Here's how the part is built. I have some questions about the finished solid (model axes, mm). Round coordinates to 2 decimals unless told otherwise and drop trailing zeros. Order: outer loops, then holes, each group sorted by start corner. A loop starts at its lowest first (then second) coordinate and runs counter-clockwise, first axis right, second up. Notation, with made-up numbers: (-31.5, -30) -> (12.5, -30) arc R19 cw to (12.5, -22) -> close; hole circle Ø6 at (86.25, 34.5). An arc over 180 degrees is marked (long way). Answer in a Markdown table with one row per item.
```python
from build123d import *

# Parameters (mm, degrees)
SKETCH001002008_R   = 1.5
SKETCH001002008_R_2 = 2.5
SKETCH001002008_W   = 9.8
SKETCH001002008_H   = 3
SKETCH001002008_W_2 = 12.8
PAD013_DEPTH        = 3
FILLET027_R         = 3
FILLET030_R         = 10


with BuildPart() as part:
    # Sketch001002008 → Pad013 (new body)
    with BuildSketch(Plane(origin=(0, 45, -16.5), x_dir=(0, -1, 0), z_dir=(0, 0, 1))):
        Polygon((-61, -198.5), (0, -198.5), (0, -108.5), (35, -108.5), (35, 198.5), (-16, 198.5), (-16, 108.5), (-61, 108.5), (-61, 98.5), (-64, 98.5), (-64, 88.5), (-61, 88.5), (-61, -168.5), (-64, -168.5), (-64, -178.5), (-61, -178.5), align=None)
        with Locations((9.5, 194)):
            Circle(SKETCH001002008_R, mode=Mode.SUBTRACT)
        with Locations((-30.5, -194)):
            Circle(SKETCH001002008_R, mode=Mode.SUBTRACT)
        with Locations((-5.1, 182.5)):
            Circle(SKETCH001002008_R, mode=Mode.SUBTRACT)
        with Locations((-36.6, 34.5)):
            Circle(SKETCH001002008_R_2, mode=Mode.SUBTRACT)
        with Locations((21.4, 34.5)):
            Circle(SKETCH001002008_R_2, mode=Mode.SUBTRACT)
        with Locations((21.4, -14.5)):
            Circle(SKETCH001002008_R_2, mode=Mode.SUBTRACT)
        with Locations((-36.6, -14.5)):
            Circle(SKETCH001002008_R_2, mode=Mode.SUBTRACT)
        with Locations((-50.1, 97.5)):
            Circle(SKETCH001002008_R, mode=Mode.SUBTRACT)
        with Locations((-50.1, -182.5)):
            Circle(SKETCH001002008_R, mode=Mode.SUBTRACT)
        with Locations((24.9, -97.5)):
            Circle(SKETCH001002008_R, mode=Mode.SUBTRACT)
        with Locations((-50.1, 32.5)):
            Circle(SKETCH001002008_R, mode=Mode.SUBTRACT)
        with Locations((-10.1, -97.5)):
            Circle(SKETCH001002008_R, mode=Mode.SUBTRACT)
        with Locations((24.9, 77.5)):
            Circle(SKETCH001002008_R, mode=Mode.SUBTRACT)
        with Locations((-45.1, 97.5)):
            Circle(SKETCH001002008_R, mode=Mode.SUBTRACT)
        with Locations((-40.1, 97.5)):
            Circle(SKETCH001002008_R, mode=Mode.SUBTRACT)
        with Locations((24.9, 97.5)):
            Circle(SKETCH001002008_R, mode=Mode.SUBTRACT)
        with Locations((-40.1, 42.5)):
            Circle(SKETCH001002008_R, mode=Mode.SUBTRACT)
        with Locations((-52, -194)):
            Rectangle(SKETCH001002008_W, SKETCH001002008_H, mode=Mode.SUBTRACT)
        with Locations((-9, -194)):
            Rectangle(SKETCH001002008_W, SKETCH001002008_H, mode=Mode.SUBTRACT)
        with Locations((-7, 194)):
            Rectangle(SKETCH001002008_W, SKETCH001002008_H, mode=Mode.SUBTRACT)
        with Locations((26, 194)):
            Rectangle(SKETCH001002008_W, SKETCH001002008_H, mode=Mode.SUBTRACT)
        with Locations((-44.5, -38)):
            Rectangle(SKETCH001002008_W_2, SKETCH001002008_H, mode=Mode.SUBTRACT)
        with BuildLine():
            ThreePointArc((-33.6, 27.5), (-35.1, 29), (-36.6, 27.5))
            Line((-36.6, 27.5), (-36.6, -7.5))
            ThreePointArc((-36.6, -7.5), (-35.1, -9), (-33.6, -7.5))
            Line((-33.6, 27.5), (-33.6, -7.5))
        make_face(mode=Mode.SUBTRACT)
        with BuildLine():
            ThreePointArc((-23.6, 32.5), (-25.1, 34), (-26.6, 32.5))
            Line((-26.6, 32.5), (-26.6, -12.5))
            ThreePointArc((-26.6, -12.5), (-25.1, -14), (-23.6, -12.5))
            Line((-23.6, 32.5), (-23.6, -12.5))
        make_face(mode=Mode.SUBTRACT)
        with BuildLine():
            ThreePointArc((-13.6, 32.5), (-15.1, 34), (-16.6, 32.5))
            Line((-16.6, 32.5), (-16.6, -12.5))
            ThreePointArc((-16.6, -12.5), (-15.1, -14), (-13.6, -12.5))
            Line((-13.6, 32.5), (-13.6, -12.5))
        make_face(mode=Mode.SUBTRACT)
        with BuildLine():
            ThreePointArc((1.4, 32.5), (-0.1, 34), (-1.6, 32.5))
            Line((-1.6, 32.5), (-1.6, -12.5))
            ThreePointArc((-1.6, -12.5), (-0.1, -14), (1.4, -12.5))
            Line((1.4, 32.5), (1.4, -12.5))
        make_face(mode=Mode.SUBTRACT)
        with BuildLine():
            ThreePointArc((11.4, 32.5), (9.9, 34), (8.4, 32.5))
            Line((8.4, 32.5), (8.4, -12.5))
            ThreePointArc((8.4, -12.5), (9.9, -14), (11.4, -12.5))
            Line((11.4, 32.5), (11.4, -12.5))
        make_face(mode=Mode.SUBTRACT)
        with BuildLine():
            ThreePointArc((21.4, 27.5), (19.9, 29), (18.4, 27.5))
            Line((18.4, 27.5), (18.4, -7.5))
            ThreePointArc((18.4, -7.5), (19.9, -9), (21.4, -7.5))
            Line((21.4, 27.5), (21.4, -7.5))
        make_face(mode=Mode.SUBTRACT)
    extrude(amount=-PAD013_DEPTH)

    # Fillet027
    fillet027_edges = [part.edges().sort_by_distance(p)[0] for p in [
        (-198.5, 45, -18),
        (198.5, 10, -18),
        (198.5, 61, -18),
    ]]
    fillet(fillet027_edges, radius=FILLET027_R)

    # Fillet030
    fillet030_edges = [part.edges().sort_by_distance(p)[0] for p in [
        (-108.5, 45, -18),
        (-108.5, 10, -18),
        (108.5, 61, -18),
    ]]
    fillet(fillet030_edges, radius=FILLET030_R)


solid = part.part
```
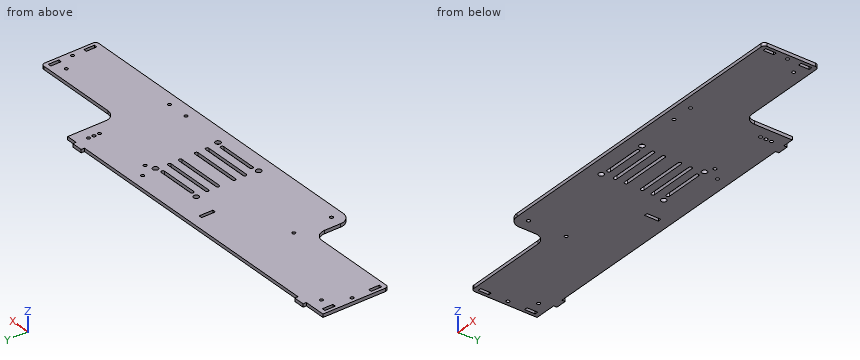
1. Suppose I cut it at A-A on z = -17.35. State how many separate pieces and enclosed holes the cut face has, then the cut area to 3 significant figures.
Numbers:
| item | result |
|---|---|
| separate pieces | 1 |
| enclosed holes | 28 |
| area | 29,900 mm2 |
2. Suppose I cut it at B-B on x = -164.5. Write out the boundary of the cut face in (y, z).
Numbers:
| item | result |
|---|---|
| outline | (45, -19.5) -> (106, -19.5) -> (106, -16.5) -> (45, -16.5) -> close |
3. Please list where these lines run through material, in increasing order: line 1 along Y through (x, z) = (-97.5, -18.7); line 2 along X through (y, z) = (95.1, -17.25); line 3 along Y through (x, z) = (97.5, -17.7).
Numbers:
| item | result |
|---|---|
| line 1 | y = 10 to 18.6, 21.6 to 53.6, 56.6 to 106 |
| line 2 | x = -198.5 to -195.5, -192.5 to -184, -181 to -39.5, -36.5 to 31, 34 to 96, 99 to 108.5 |
| line 3 | y = 10 to 18.6, 21.6 to 83.6, 86.6 to 88.6, 91.6 to 93.6, 96.6 to 109 |
4. Suppose I cut it at C-C on x = 158.5. Write out the boundary of the cut face in (y, z).
Numbers:
| item | result |
|---|---|
| outline | (10, -19.5) -> (61, -19.5) -> (61, -16.5) -> (10, -16.5) -> close |
5. For pin 1 Ø0.9 at (x, z) = (13.5, -17.5) entering from +Y; pin 2 Ø3 at (x, y) = (34.5, 23.6) entering from +Z; pin 3 Ø0.9 at (x, z) = (-174, -18.5) entering from -Y, each with a flat end and sliding along its axis, tell me the tip position at first contact or that it passes through.
Numbers:
| item | result |
|---|---|
| pin 1 | stops at y = 106 |
| pin 2 | passes through |
| pin 3 | stops at y = 45 |
